Source: CAD feature listing. Evaluate the final solid. Frame: model axes, mm. A direction names the side the tool comes from. Round coordinates to 2 decimals unless told otherwise and drop trailing zeros. Order: outer loops, then holes, each group sorted by start corner. A loop starts at its lowest first (then second) coordinate and runs counter-clockwise, first axis right, second up.
```python
from build123d import *

# Parameters (mm, degrees)
SKETCH_1_R           = 60
SKETCH_1_R_2         = 40
EXTRUDE_1_DEPTH      = 20
SKETCH_2_R           = 60
EXTRUDE_4_DEPTH      = 5
EXTRUDE_5_REACH      = 160.459
EXTRUDE_5_END_RADIUS = 60
EXTRUDE_START        = -70
SKETCH_3_W           = 40
SKETCH_3_H           = 40
SKETCH_4_R           = 2.5
CUT_EXTRUDE_1_DEPTH  = 5
EXTRUDE_START_2      = 10.5
SKETCH_5_R           = 40
EXTRUDE_6_DEPTH      = 10.5
EXTRUDE_7_DEPTH      = 10


with BuildPart() as part:
    # 草图1 → 凸台-拉伸1 (new body)
    with BuildSketch(Plane(origin=(0, 0, 0), x_dir=(1, 0, 0), z_dir=(0, 1, 0))):
        with Locations(Location((0, 0, 0), (0, 0, 270))):
            Circle(SKETCH_1_R)
        with Locations(Location((0, 0, 0), (0, 0, 270))):
            Circle(SKETCH_1_R_2, mode=Mode.SUBTRACT)
    extrude(amount=EXTRUDE_1_DEPTH)

    # 草图2 → 凸台-拉伸4 (add)
    with BuildSketch(Plane(origin=(0, 20, 0), x_dir=(1, 0, 0), z_dir=(0, 1, 0))):
        with Locations(Location((0, 0, 0), (0, 0, 270))):
            Circle(SKETCH_2_R)
    extrude(amount=EXTRUDE_4_DEPTH)

    # 凸台-拉伸5: up to this cylinder (the profile starts outside it)
    extrude_5_end = Plane(origin=(0, 12.5, 0), z_dir=(0, -1, 0)) * Cylinder(EXTRUDE_5_END_RADIUS, 441.918, mode=Mode.PRIVATE)
    # 草图3 → 凸台-拉伸5 (add, up to the surface)
    with BuildSketch(Plane(origin=(0, 0, 0), x_dir=(0, 0, -1), z_dir=(1, 0, 0)).offset(EXTRUDE_START), mode=Mode.PRIVATE) as extrude_5_sk1:
        with Locations((0, 12.5)):
            Rectangle(SKETCH_3_W, SKETCH_3_H)
    extrude_5_tool1 = extrude(extrude_5_sk1.sketch, amount=EXTRUDE_5_REACH, mode=Mode.PRIVATE) - extrude_5_end
    add(extrude_5_tool1.solids().sort_by_distance((-70, 12.5, 0))[0])

    # 草图4 → 切除-拉伸1 (cut)
    with BuildSketch(Plane.ZY.offset(70)):
        with Locations((-15, 27.5)):
            Circle(SKETCH_4_R)
        with Locations((15, 27.5)):
            Circle(SKETCH_4_R)
        with Locations((15, -2.5)):
            Circle(SKETCH_4_R)
        with Locations((-15, -2.5)):
            Circle(SKETCH_4_R)
    extrude(amount=-CUT_EXTRUDE_1_DEPTH, mode=Mode.SUBTRACT)

    # 草图5 → 凸台-拉伸6 (add)
    with BuildSketch(Plane.XZ.offset(EXTRUDE_START_2)):
        with BuildLine():
            ThreePointArc((-56.568542495, 20), (-60, 0), (-56.568542495, -20))
            ThreePointArc((-56.568542495, -20), (60, 0), (-56.568542495, 20))
        make_face()
        with Locations(Location((0, 0, 0), (0, 0, 270))):
            Circle(SKETCH_5_R, mode=Mode.SUBTRACT)
    extrude(amount=-EXTRUDE_6_DEPTH)

    # 草图6 → 凸台-拉伸7 (add)
    with BuildSketch(Plane(origin=(0, 25, 0), x_dir=(1, 0, 0), z_dir=(0, 1, 0))):
        with BuildLine():
            ThreePointArc((-56.568542495, 20), (-60, 0), (-56.568542495, -20))
            ThreePointArc((-56.568542495, -20), (60, 0), (-56.568542495, 20))
        make_face()
    extrude(amount=EXTRUDE_7_DEPTH)


solid = part.part
```
1. Section D-D on y = 22.5. Return loops of the section in (x, z).
2. Section B-B on y = -2.5. Return loops of the section in (x, z).
3. Section C-C on x = 0. Return loops of the section in (y, z), plus the area to 3 significant figures.
4. Line query: line 1 along Y through (x, z) = (-66, 15); line 2 along X through (y, z) = (15, 0); line 3 along X through (y, z) = (-5.5, -6). Output: solid intervals per line, ascending.
5. Pull-direction query (Z, two-part tool) for faces 6 (the face through (-65, -7.5, 0)), 7 (the face through (-67.5, -2.4, 12.5)), 8 (the face through (-63, 12, -20)); classes: released by +Z, released by -Z, zero draft, split by the parting line, or undercut.
6. Access query for faces 1 (the face through (-65, -2, -15)), 2 (the face through (1, 20, -1)), 3 (the face through (-70, 13, 0)), 4 (the face through (-1, 35, -1)), 5 (the face through (-63, 12, 20)). Directions: +Z, -Z, +X, -X, +Y, -Y. A direction counts if a zero-diameter tool reaches every point of the face in a straight line with its end or side. Return the directions, or none.
7. First-contact query: pin 1 (4.5 mm diameter, centred on y = 27.5, z = -15, fed in from +X); pin 2 (3 mm diameter, centred on y = -2.5, z = -15, fed in from +X); pin 3 (24 mm diameter, centred on x = 9, z = 2, fed in from -Y). Flat tips, straight axial feed; report the tip coordinate or a pass-through.
8. Section A-A on z = 0. Return loops of the section in (x, y), plus the area to 3 significant figures.
Result:
1. outline: (-70, -20) - (-56.57, -20) arc R60 ccw (long way) to (-56.57, 20) - (-70, 20) - close
2. outline: (-70, -20) - (-56.57, -20) arc R60 ccw (long way) to (-56.57, 20) - (-70, 20) - (-70, 17.5) - (-65, 17.5) - (-65, 12.5) - (-70, 12.5) - (-70, -12.5) - (-65, -12.5) - (-65, -17.5) - (-70, -17.5) - close; hole circle Ø80 at (0, 0)
3. outline: (-10.5, -60) - (35, -60) - (35, 60) - (-10.5, 60) - (-10.5, 40) - (20, 40) - (20, -40) - (-10.5, -40) - close
3. area: 3,020 mm2
4. line 1: y = -7.5 to -5, 0 to 25, 30 to 32.5
4. line 2: x = -70 to -40, 40 to 60
4. line 3: x = -70 to -39.55, 39.55 to 59.7
5. face 6: zero draft
5. face 7: undercut
5. face 8: released by -Z
6. face 1: -X
6. face 2: -Y
6. face 3: +Z, -Z, -X, +Y, -Y
6. face 4: +Z, -Z, +X, -X, +Y
6. face 5: +Z, -X, +Y, -Y
7. pin 1: stops at x = 58.63
7. pin 2: stops at x = 58.46
7. pin 3: stops at y = 20
8. outline: (-70, -7.5) - (-60, -7.5) - (-60, -10.5) - (-40, -10.5) - (-40, 20) - (40, 20) - (40, -10.5) - (60, -10.5) - (60, 35) - (-60, 35) - (-60, 32.5) - (-70, 32.5) - close
8. area: 3,420 mm2
